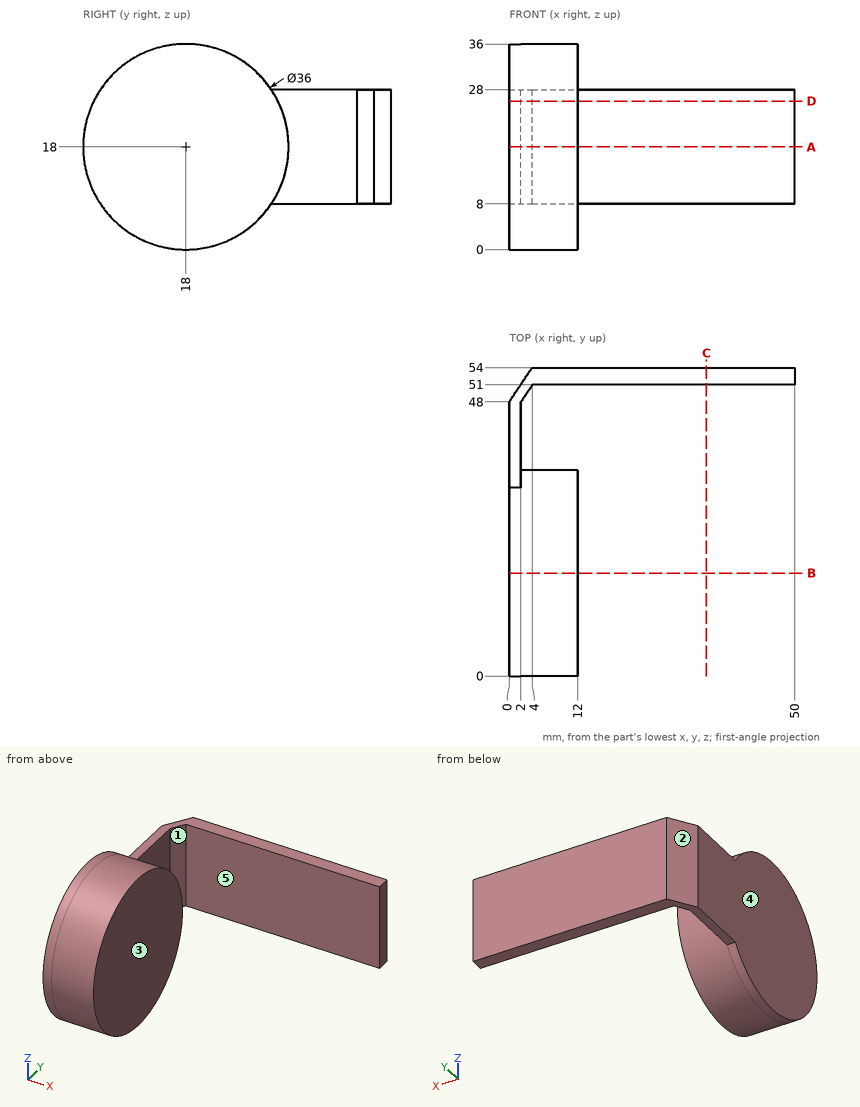
Verification items for this drawing (mm, ordinates from the low corner). A direction names the side the tool comes from. Give positions to 0.01 mm unless a question says otherwise; leave off trailing zeros. Loops run counter-clockwise (first coordinate to the right, second up) from the corner with the lowest first, then second, coordinate; pieces in that order, holes last. Notation, with made-up numbers: M -21,-24 L 10,-24 A19 ccw 10,-19 Z; hole C 47,63 d9. An arc over 180 degrees is marked long. Return JSON: item names as keys, results as strings. Group by question number.
1. Go/stop test with flat-tipped pins: pin 1 (4 mm diameter, centred on y = 30, z = 18.5, fed in from +X); pin 2 (10 mm diameter, centred on x = 29, z = 17, fed in from -Y); pin 3 (6.5 mm diameter, centred on x = 20.5, y = 48.5, fed in from +Z). Record where each tip stops, or that it passes through.
2. Cross-section at A-A on z = 18. Record the boundary of the cut face in (x, y), plus the area to 3 significant figures.
3. Cross-section at C-C on x = 34.5. Record the boundary of the cut face in (y, z).
4. Thickness scan on L1, parallel to X at y = 14, z = 24.5; L2, parallel to Y at x = 34, z = 13; L3, parallel to Y at x = 6, z = 25. Record the ranges inside material, lowest first.
5. Mould release check, pull along Y, two halves, no side actions. Record for the marked faces 1, 2 and 3: released by +Y, released by -Y, zero draft, split by the parting line, or undercut.
6. Cross-section at B-B on y = 18. Record the boundary of the cut face in (x, z).
7. Tool access check on the marked faces 4 and 5. Record the directions out of +Z, -Z, +X, -X, +Y, -Y that give a thin tool (end or side, any length) a straight path to the whole face; none if there is none.
8. Cross-section at D-D on z = 26. Record the boundary of the cut face in (x, y), plus the area to 3 significant figures.
Return value:
{
 "1": {"pin 1": "x = 12", "pin 2": "y = 51", "pin 3": "z = 28"},
 "2": {"outline": "M 0,0 L 12,0 L 12,36 L 2,36 L 2,48 L 4,51 L 50,51 L 50,54 L 4,54 L 0,48 Z", "area": "603 mm^2"},
 "3": {"outline": "M 51,8 L 54,8 L 54,28 L 51,28 Z"},
 "4": {"L1": "0 to 12", "L2": "51 to 54", "L3": "1.42 to 34.58, 51 to 54"},
 "5": {"face 1": "undercut", "face 2": "released by +Y", "face 3": "zero draft"},
 "6": {"outline": "M 0,0 L 12,0 L 12,36 L 0,36 Z"},
 "7": {"face 4": "+Z, -Z, -X, +Y, -Y", "face 5": "+Z, -Z, +X"},
 "8": {"outline": "M 0,1.88 L 12,1.88 L 12,34.12 L 2,34.12 L 2,48 L 4,51 L 50,51 L 50,54 L 4,54 L 0,48 Z", "area": "562 mm^2"}
}
